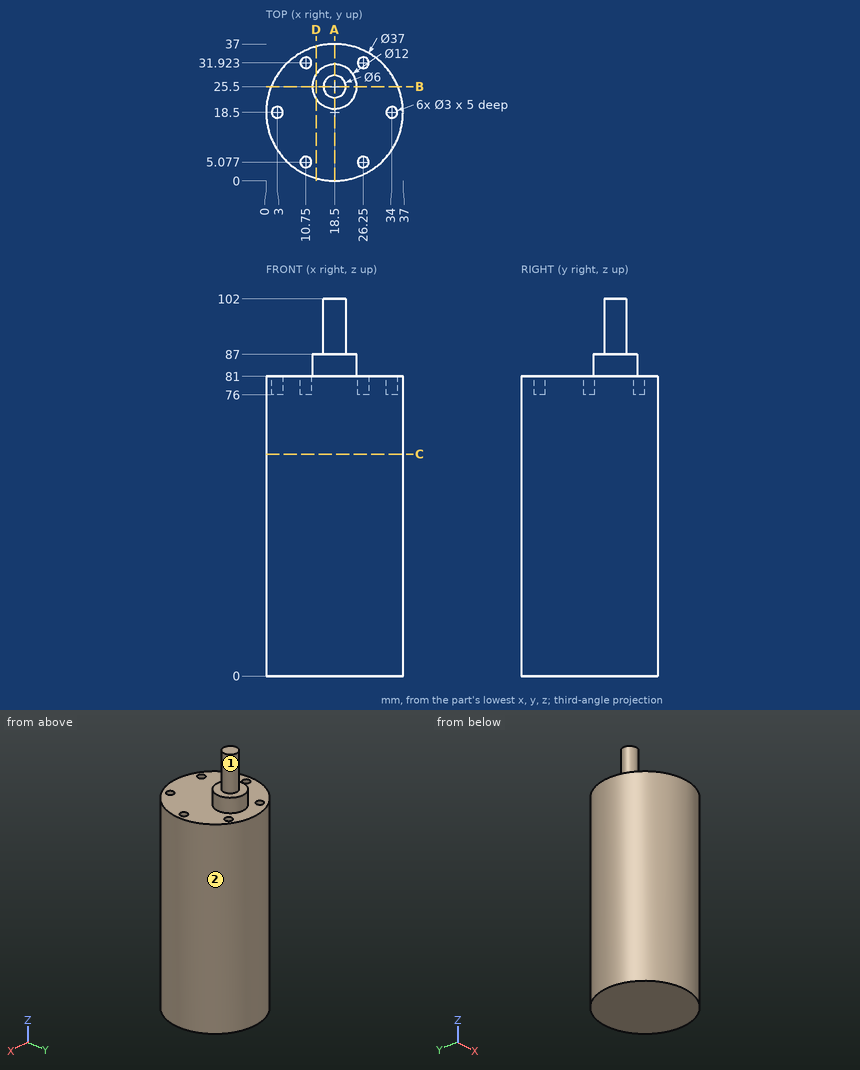
Source: three-view drawing plus pictorial views. Frame: mm from the lowest corner of the part. A direction names the side the tool comes from. Coordinates: 2 decimals unless noted, no trailing zeros. Loops run counter-clockwise (first coordinate to the right, second up) from the corner with the lowest first, then second, coordinate; pieces in that order, holes last. Notation, with made-up numbers: M 54.25,35 L 103.25,35 A32 ccw 103.25,73 Z; hole C 66,77.5 d10. An arc over 180 degrees is marked long. Use CSV: the item, a comma, the result in double quotes.
(1) Cut plane B-B on y = 25.5. Return loops of the section in (x, z) (1 decimal).
Answers follow:
outline,"M 1.4,0 L 35.6,0 L 35.6,81 L 24.5,81 L 24.5,87 L 21.5,87 L 21.5,102 L 15.5,102 L 15.5,87 L 12.5,87 L 12.5,81 L 1.4,81 Z"
(2) Cut plane C-C on z = 60. Return loops of the section in (x, y).
Answers follow:
outline,"C 18.5,18.5 d37"
(3) Reachability of the marked faces 1 and 2 from +Z, -Z, +X, -X, +Y, -Y: full face, straight path, thin tool, end or side. Return the list, or none.
Answers follow:
face 1,"+Z"
face 2,"+Z, -Z"
(4) Line query: line 1 (Y direction, x = 10, z = 78) (1 decimal); line 2 (Y direction, x = 10.75, z = 78.1); line 3 (Z direction, x = 2, y = 18.5). Output: solid intervals per line, ascending. Write a range as [from, to].
Answers follow:
line 1,"[2.1, 3.8], [6.4, 30.6], [33.2, 34.9]"
line 2,"[1.7, 3.58], [6.58, 30.42], [33.42, 35.3]"
line 3,"[0, 76]"
(5) Cut plane D-D on x = 13.5. Return loops of the section in (y, z), and give its area (3 significant figures).
Answers follow:
outline,"M 0.69,0 L 36.31,0 L 36.31,81 L 28.82,81 L 28.82,87 L 22.18,87 L 22.18,81 L 0.69,81 Z"
area,"2,930 mm²"
(6) Contact query for flat-ended pins moving along their axis: pin 1 (1 mm diameter, centred on x = 28.5, z = 56.5, fed in from +Y) (1 decimal); pin 2 (6 mm diameter, centred on y = 29.5, z = 12, fed in from -X); pin 3 (2.5 mm diameter, centred on x = 10.5, y = 5.5, fed in from +Z). Output: stop coordinate, or through.
Answers follow:
pin 1,"y = 34.4"
pin 2,"x = 1.82"
pin 3,"z = 81"
(7) Cut plane A-A on x = 18.5. Return loops of the section in (y, z).
Answers follow:
outline,"M 0,0 L 37,0 L 37,81 L 31.5,81 L 31.5,87 L 28.5,87 L 28.5,102 L 22.5,102 L 22.5,87 L 19.5,87 L 19.5,81 L 0,81 Z"
